Solid Edge part; units mm, degrees
sketch "Sketch1" plane through (0, 0, 0) normal (0, -1, 0) x (1, 0, 0)
  circle A0 centre (0, -7) radius 4.2
  circle A1 centre (0, 7) radius 4.2
extrude "Protrusion1" add sketch "Sketch1" along normal blind 7.8
sketch "Sketch2" plane through (0, 0, -7) normal (0, 1, 0) x (-1, 0, 0)
  line L0 (8, -6.25) -> (-8, -6.25)
  line L1 (-8, -6.25) -> (-8, 20.25)
  line L2 (-8, 20.25) -> (8, 20.25)
  line L3 (8, 20.25) -> (8, -6.25)
extrude "ExtrudedProtrusion_2" add sketch "Sketch2" along normal blind 14.5
sketch "Sketch3" plane through (0, 7.25, -13.25) normal (0, 0, -1) x (1, 0, 0)
  line L0 (-6.4, 1.25) -> (-6.4, -1.75)
  line L1 (-6.4, -1.75) -> (-8.1, -1.75)
  line L2 (-8.1, -1.75) -> (-8.1, 1.25)
  line L3 (-8.1, 1.25) -> (-6.4, 1.25)
  circle A0 centre (4, -4.25) radius 0.6
  circle A1 centre (-4, -3) radius 0.6
  circle A2 centre (0, 0.25) radius 0.6
  line L4 (6.4, 1.25) -> (8.1, 1.25)
  line L5 (8.1, 1.25) -> (8.1, -1.75)
  line L6 (8.1, -1.75) -> (6.4, -1.75)
  line L7 (6.4, -1.75) -> (6.4, 1.25)
extrude "ExtrudedProtrusion_3" add sketch "Sketch3" along normal blind 5.1
sketch "Sketch4" plane through (0, 0, 0) normal (0, -1, 0) x (1, 0, 0)
  line L0 (8, -0.6633) -> (8, -7.62)
  line L1 (8, -7.62) -> (10.2225, -3.3861)
  arc A0 (10.2225, 3.3861) -> (10.2225, -3.3861) centre (9, 0) cw
  line L2 (10.2225, 3.3861) -> (8, 7.62)
  line L3 (8, 7.62) -> (8, 0.6633)
  arc A1 (8, 0.6633) -> (8, -0.6633) centre (9, 0) cw
extrude "ExtrudedProtrusion_4" add sketch "Sketch4" against normal blind 2
The model under review builds one solid part; all positions refer to its coordinate system, in mm. A direction names the side the tool comes from. Round coordinates to 2 decimals unless told otherwise and drop trailing zeros. Loops run counter-clockwise (first coordinate to the right, second up) from the corner with the lowest first, then second, coordinate; pieces in that order, holes last. Notation, with made-up numbers: M 46,55 L 80,55 A15 ccw 80,68 Z; hole C 68,60.25 d11. An arc over 180 degrees is marked long. Put each result on its own line as item: value.
Q1. For pin 1 (1.9 mm diameter, centred on x = 7, z = -16, fed in from +Y); pin 2 (4.5 mm diameter, centred on y = 5, z = -1.5, fed in from -X); pin 3 (10 mm diameter, centred on y = 0, z = -7.5, fed in from +X); pin 4 (1 mm diameter, centred on x = 9, y = 8.5, fed in from -Z), all flat-tipped, find the tip position at first contact; note any pin that passes through.
Result set:
pin 1: stops at y = 9
pin 2: stops at x = -8
pin 3: stops at x = 11.59
pin 4: passes through
Q2. To check wall thickness, follow L1, parallel to X at y = 8.25, z = -16.5; L2, parallel to X at y = 11, z = 3; L3, parallel to Z at x = 9, y = 1.5. State the ranges of each line that lie inside material, in increasing order.
Result set:
L1: x = -8.1 to -6.4, 6.4 to 8.1
L2: x = -8 to 8
L3: z = -5.71 to -1.2, 1.2 to 5.71
Q3. Consider section D-D, the plane y = -1.75. Give the boundary of the cut face in (x, z).
Result set:
outline: C 0,-7 d8.4; C 0,7 d8.4
Q4. Consider section A-A, the plane x = 9. Give the boundary of the cut face in (y, z).
Result set:
outline: M 0,-5.71 L 2,-5.71 L 2,-1.2 L 0,-1.2 Z; M 0,1.2 L 2,1.2 L 2,5.71 L 0,5.71 Z
Q5. Consider section C-C, the plane x = 0. Give the boundary of the cut face in (y, z).
Result set:
outline: M -7.8,-11.2 L 0,-11.2 L 0,-13.25 L 6.4,-13.25 L 6.4,-18.35 L 7.6,-18.35 L 7.6,-13.25 L 14.5,-13.25 L 14.5,13.25 L 0,13.25 L 0,11.2 L -7.8,11.2 L -7.8,2.8 L 0,2.8 L 0,-2.8 L -7.8,-2.8 Z
Q6. Consider section B-B, the plane y = 11.5. Give the boundary of the cut face in (x, z).
Result set:
outline: M -8,-13.25 L 3.4,-13.25 L 3.4,-18.35 L 4.6,-18.35 L 4.6,-13.25 L 8,-13.25 L 8,13.25 L -8,13.25 Z
Q7. Machinability: for faces 1 (the flat face through (-8, 7, 0)), 2 (the flat face through (-7, 6, -16)), 3 (the flat face through (-6.4, 7, -16)), which of the approach directions +Z, -Z, +X, -X, +Y, -Y give a long, thin tool a straight path to every point of the face, cutting with its end or side? Answer none if there is none.
Result set:
face 1: +Z, -X, +Y, -Y
face 2: -Z, +X, -X, -Y
face 3: -Z, +Y, -Y
Q8. Mouldability with a two-part tool opening along X and no side actions: class faces 4 (the cylindrical face through (-0.13, 6.414, -15.764)), 5 (the cylindrical face through (-4.13, 9.664, -15.764)), 6 (the flat face through (8.1, 7, -16)) as released by +X, released by -X, zero draft, split by the parting line, or undercut.
Result set:
face 4: undercut
face 5: split by the parting line
face 6: released by +X
